from build123d import *

# Parameters (mm, degrees)
BOSS_EXTRUDE1_DEPTH = 9.525
SKETCH2_R           = 2.0955
CUT_EXTRUDE1_DEPTH  = 29.848015755


with BuildPart() as part:
    # Sketch1 → Boss-Extrude1 (new body)
    with BuildSketch(Plane.XY):
        with BuildLine():
            Line((0, 8.382), (12.363477137, 8.382))
            ThreePointArc((12.363477137, 8.382), (24.411145213, 11.134714393), (19.05, 0))
            Line((19.05, 0), (0, 0))
            Line((0, 0), (0, 0.762))
            Line((0, 0.762), (19.05, 0.762))
            ThreePointArc((19.05, 0.762), (23.622, 10.890124998), (13.001812503, 7.62))
            Line((13.001812503, 7.62), (0, 7.62))
            Line((0, 7.62), (0, 8.382))
        make_face()
    extrude(amount=BOSS_EXTRUDE1_DEPTH)

    # Sketch2 → Cut-Extrude1 (cut, through all)
    with BuildSketch(Plane(origin=(0, 8.382, 0), x_dir=(1, 0, 0), z_dir=(0, 1, 0))):
        with Locations(Location((4.7625, -4.7625, 0), (0, 0, 270))):
            Circle(SKETCH2_R)
        with BuildLine():
            Line((0, 0), (0, -4.7625))
            ThreePointArc((0, -4.7625), (1.394903955, -1.394903955), (4.7625, 0))
            Line((4.7625, 0), (0, 0))
        make_face()
        with BuildLine():
            Line((0, -9.525), (4.7625, -9.525))
            ThreePointArc((4.7625, -9.525), (1.394903955, -8.130096045), (0, -4.7625))
            Line((0, -4.7625), (0, -9.525))
        make_face()
    extrude(amount=-CUT_EXTRUDE1_DEPTH, mode=Mode.SUBTRACT)


solid = part.part
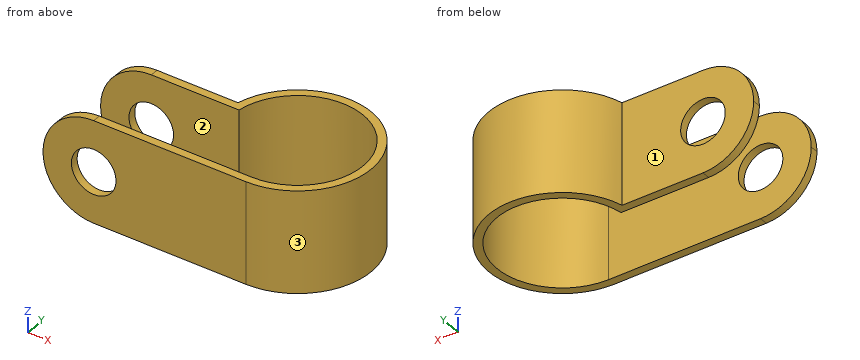
Geometry check sheet. Reference: the model listing, model coordinates, mm. Face numbers are marked on the shaded views. A direction names the side the tool comes from. Round coordinates to 2 decimals unless told otherwise and drop trailing zeros. Loops run counter-clockwise (first coordinate to the right, second up) from the corner with the lowest first, then second, coordinate; pieces in that order, holes last. Notation, with made-up numbers: (82, -12) - (109, -12) arc R24 ccw to (109, 21) - close; hole circle Ø4 at (50, 84.25). An arc over 180 degrees is marked (long way). Answer as CSV lines item,"result".
(1) Cross-section at C-C, the plane z = 5.5. Enter the section's corners in (x, y), and give its area (3 significant figures).
Output values:
outline,"(0.06, 0) - (2.8, 0) - (2.8, 0.76) - (0.06, 0.76) - close; (0.06, 7.62) - (2.8, 7.62) - (2.8, 8.38) - (0.06, 8.38) - close; (6.72, 0) - (19.05, 0) arc R6.86 ccw (long way) to (12.36, 8.38) - (6.72, 8.38) - (6.72, 7.62) - (13, 7.62) arc R6.1 cw (long way) to (19.05, 0.76) - (6.72, 0.76) - close"
area,"40.5 mm²"
(2) Cross-section at B-B, the plane x = 5.75. Enter the section's corners in (y, z) (3 decimals), and give its area (3 significant figures).
Output values:
outline,"(0, 0) - (0.762, 0) - (0.762, 2.914) - (0, 2.914) - close; (0, 6.611) - (0.762, 6.611) - (0.762, 9.525) - (0, 9.525) - close; (7.62, 0) - (8.382, 0) - (8.382, 2.914) - (7.62, 2.914) - close; (7.62, 6.611) - (8.382, 6.611) - (8.382, 9.525) - (7.62, 9.525) - close"
area,"8.88 mm²"
(3) Cross-section at A-A, the plane y = 9.75. Enter the section's corners in (x, z) (3 decimals), and give its area (3 significant figures).
Output values:
outline,"(12.832, 0) - (13.684, 0) - (13.684, 9.525) - (12.832, 9.525) - close; (24.416, 0) - (25.268, 0) - (25.268, 9.525) - (24.416, 9.525) - close"
area,"16.2 mm²"
(4) Cross-section at D-D, the plane x = 23.75. Enter the section's corners in (y, z) (3 decimals), and give its area (3 significant figures).
Output values:
outline,"(1.864, 0) - (2.976, 0) - (2.976, 9.525) - (1.864, 9.525) - close; (10.74, 0) - (11.852, 0) - (11.852, 9.525) - (10.74, 9.525) - close"
area,"21.2 mm²"
(5) Set-up check for the marked faces 1, 2 and 3: record each of +Z, -Z, +X, -X, +Y, -Y from which the full face is reachable in a straight line by a thin tool's end or side.
Output values:
face 1,"+Z, -Z, -X, +Y"
face 2,"+Z, -Z, -X"
face 3,"+Z, -Z"
(6) Material ranges on line 1 along X through (y, z) = (8, 4); line 2 along Y through (x, z) = (2, 4.5); line 3 along Y through (x, z) = (16.5, 3.5), recorded low to high.
Output values:
line 1,"x = 0.06 to 2.81, 6.71 to 13.06, 25.04 to 25.81"
line 2,"y = 0 to 0.76, 7.62 to 8.38"
line 3,"y = 0 to 0.76, 12.4 to 13.22"
(7) Depth check by flat-ended pin: pin 1 Ø3 at (y, z) = (9.5, 1.5) entering from -X; pin 2 Ø1.5 at (x, z) = (4, 3.5) entering from +Y; pin 3 Ø5 at (x, z) = (12.5, 4.5) entering from +Y. Enter the tip coordinate at first touch or a pass-through.
Output values:
pin 1,"stops at x = 0.57"
pin 2,"stops at y = 8.38"
pin 3,"stops at y = 12.39"
